from build123d import *

# Parameters (mm, degrees)
SKETCH1_R           = 25.4
BOSS_EXTRUDE1_DEPTH = 3
CUT_EXTRUDE1_DEPTH  = 5
SKETCH3_R           = 2
CUT_EXTRUDE2_DEPTH  = 5


with BuildPart() as part:
    # Sketch1 → Boss-Extrude1 (new body)
    with BuildSketch(Plane(origin=(0, 0, 0), x_dir=(1, 0, 0), z_dir=(0, 1, 0))):
        with Locations(Location((0, 0, 0), (0, 0, 270))):
            Circle(SKETCH1_R)
    extrude(amount=BOSS_EXTRUDE1_DEPTH)

    # Sketch2 → Cut-Extrude1 (cut)
    with BuildSketch(Plane(origin=(0, 3, 0), x_dir=(1, 0, 0), z_dir=(0, 1, 0))):
        with BuildLine():
            Line((2.854423328, 0.923183333), (0, 3))
            ThreePointArc((0, 3), (-2.121320344, -2.121320344), (3, 0))
            ThreePointArc((3, 0), (2.963382357, 0.467295419), (2.854423328, 0.923183333))
        make_face()
    extrude(amount=-CUT_EXTRUDE1_DEPTH, mode=Mode.SUBTRACT)

    # Sketch3 → Cut-Extrude2 (cut)
    with BuildSketch(Plane(origin=(0, 3, 0), x_dir=(1, 0, 0), z_dir=(0, 1, 0))):
        with Locations(Location((0, 17, 0), (0, 0, 270))):
            Circle(SKETCH3_R)
        with Locations(Location((14.722431864, -8.5, 0), (0, 0, 270))):
            Circle(SKETCH3_R)
        with Locations(Location((-14.722431864, -8.5, 0), (0, 0, 270))):
            Circle(SKETCH3_R)
    extrude(amount=-CUT_EXTRUDE2_DEPTH, mode=Mode.SUBTRACT)


solid = part.part
Model file for the job. Use its own axes, mm. Give positions to 0.01 mm unless a question says otherwise; leave off trailing zeros. Order: outer loops, then holes, each group sorted by start corner. A loop starts at its lowest first (then second) coordinate and runs counter-clockwise, first axis right, second up. Notation, with made-up numbers: (46, 35) -> (80, 35) arc R16 cw to (80, 44) -> close; hole circle Ø11 at (-30.75, 32.5). An arc over 180 degrees is marked (long way). Use CSV: the item, a comma, the result in double quotes.
1. Drill centre lines: line 1 along X through (y, z) = (1.5, 7); line 2 along X through (y, z) = (1.05, 8); line 3 along Z through (x, y) = (15.5, 2). Where is each one in solid material? Low to high. Write a range as from..to.
Outcome:
line 1,"-24.42..-16.05, -13.4..13.4, 16.05..24.42"
line 2,"-24.11..-16.66, -12.79..12.79, 16.66..24.11"
line 3,"-20.12..6.66, 10.34..20.12"
2. Mould opens along X. For faces 1 (the cylindrical face through (-15.456, 1.479, -20.157)), 2 (the flat face through (1.447, 1.521, -1.947)), 3 (the flat face through (0, 3, 5)) say: +X half, -X half, draft (parallel to the pull), parting line (faces both ways), or undercut.
Outcome:
face 1,"parting line"
face 2,"undercut"
face 3,"draft"
3. Band-saw the part on A-A, the plane z = 8.5. Give the cut face in (x, y), then the cut area to 3 significant figures.
Outcome:
outline,"(-23.94, 0) -> (-16.72, 0) -> (-16.72, 3) -> (-23.94, 3) -> close; (-12.72, 0) -> (12.72, 0) -> (12.72, 3) -> (-12.72, 3) -> close; (16.72, 0) -> (23.94, 0) -> (23.94, 3) -> (16.72, 3) -> close"
area,"120 mm²"
4. Band-saw the part on B-B, the plane z = -17. Give the cut face in (x, y), then the cut area to 3 significant figures.
Outcome:
outline,"(-18.87, 0) -> (-2, 0) -> (-2, 3) -> (-18.87, 3) -> close; (2, 0) -> (18.87, 0) -> (18.87, 3) -> (2, 3) -> close"
area,"101 mm²"
5. Band-saw the part on D-D, the plane x = -21. Give the cut face in (y, z).
Outcome:
outline,"(0, -14.29) -> (3, -14.29) -> (3, 14.29) -> (0, 14.29) -> close"
6. Drop flat-ended pins along their axis: pin 1 (2.5 mm diameter, centred on x = 0, z = -17, fed in from -Y); pin 2 (1 mm diameter, centred on y = 2.5, z = -14.5, fed in from -X); pin 3 (1 mm diameter, centred on y = 2.5, z = -15.5, fed in from -X). Give the stop position or say it passes through.
Outcome:
pin 1,"through"
pin 2,"x = -21.19"
pin 3,"x = -20.5"
7. Band-saw the part on C-C, the plane y = 1. Give the cut face in (x, z), then the cut area to 3 significant figures.
Outcome:
outline,"circle Ø50.8 at (0, 0); hole circle Ø4 at (-14.72, 8.5); hole circle Ø4 at (0, -17); hole (0, -3) -> (2.85, -0.92) arc R3 ccw (long way) to start; hole circle Ø4 at (14.72, 8.5)"
area,"1,960 mm²"
